Here's how the part is built. I have some questions about the finished solid (model axes, mm). A direction names the side the tool comes from. Give positions to 0.01 mm unless a question says otherwise; leave off trailing zeros. Write each loop counter-clockwise with the first axis right and the second up, starting at its lowest first coordinate (ties: lowest second). Pieces come first, ordered by that corner, then holes. Notation, with made-up numbers: (85.25, 0.25) -> (91.25, 0.25) arc R30 ccw to (91.25, 37.25) -> close; hole circle Ø6 at (59, 61). An arc over 180 degrees is marked (long way). Return JSON: item names as keys, results as strings.
from build123d import *

# Parameters (mm, degrees)
F0_W     = 38.1
F0_H     = 25.4
F1_DEPTH = 12.7
F2_W     = 34.925
F2_H     = 22.225
F3_DEPTH = 1.5875
F4_R     = 0.762
F5_R     = 0.254


with BuildPart() as f1:
    # F0 (on Top) → F1 (new body)
    with BuildSketch(Plane.XY):
        Rectangle(F0_W, F0_H)
    extrude(amount=F1_DEPTH)

    # F2 (on face) → F3 (cut)
    with BuildSketch(Plane.XY.offset(12.7)):
        Rectangle(F2_W, F2_H)
    extrude(amount=-F3_DEPTH, mode=Mode.SUBTRACT)

    # F4
    f4_edges = [f1.edges().sort_by_distance(p)[0] for p in [
        (-19.05, -12.7, 6.35),
        (-19.05, 12.7, 6.35),
        (19.05, 12.7, 6.35),
        (19.05, -12.7, 6.35),
    ]]
    fillet(f4_edges, radius=F4_R)

    # F5
    f5_edges = [f1.edges().sort_by_distance(p)[0] for p in [
        (0, 12.7, 12.7),
        (18.826815, 12.476815, 12.7),
        (-18.826815, 12.476815, 12.7),
        (19.05, 0, 12.7),
        (-19.05, 0, 12.7),
        (18.826815, -12.476815, 12.7),
        (-18.826815, -12.476815, 12.7),
        (0, -12.7, 12.7),
        (0, 11.1125, 12.7),
        (-17.4625, 0, 12.7),
        (0, -11.1125, 12.7),
        (17.4625, 0, 12.7),
    ]]
    fillet(f5_edges, radius=F5_R)


solid = f1.part
1. Which directions (+Z, -Z, +X, -X, +Y, -Y) give clear straight access to the entire face, cutting with the end or side of a thin tool? Please do faces 1 (the face through (0, 0, 0)), 2 (the face through (0, 11.112, 12)).
Taken from the geometry:
{"face 1": "-Z, +X, -X, +Y, -Y", "face 2": "+Z"}
2. Suppose I cut it at A-A, the plane y = 2.25. List the corners of the cut face in (x, z) for me, and give its area (3 significant figures).
Taken from the geometry:
{"outline": "(-19.05, 0) -> (19.05, 0) -> (19.05, 12.45) arc R0.25 ccw to (18.8, 12.7) -> (17.72, 12.7) arc R0.25 ccw to (17.46, 12.45) -> (17.46, 11.11) -> (-17.46, 11.11) -> (-17.46, 12.45) arc R0.25 ccw to (-17.72, 12.7) -> (-18.8, 12.7) arc R0.25 ccw to (-19.05, 12.45) -> close", "area": "428 mm²"}
3. Suppose I cut it at B-B, the plane z = 12. List the corners of the cut face in (x, y) for me.
Taken from the geometry:
{"outline": "(-19.05, -11.94) arc R0.76 ccw to (-18.29, -12.7) -> (18.29, -12.7) arc R0.76 ccw to (19.05, -11.94) -> (19.05, 11.94) arc R0.76 ccw to (18.29, 12.7) -> (-18.29, 12.7) arc R0.76 ccw to (-19.05, 11.94) -> close; hole (-17.46, -11.11) -> (17.46, -11.11) -> (17.46, 11.11) -> (-17.46, 11.11) -> close"}
4. For pin 1 Ø6.5 at (x, y) = (-7, -0.5) entering from +Z, with a flat end and sliding along its axis, tell me the tip position at first contact or that it passes through.
Taken from the geometry:
{"pin 1": "stops at z = 11.11"}
5. If I drill on line 1 (Y direction, x = 2, z = 12); line 2 (X direction, y = -1.75, z = 11.5); line 3 (Z direction, x = 9, y = 8.25), over which ranges is the centre line in solid material (lowest first)? Write a range as [from, to].
Taken from the geometry:
{"line 1": "y = [-12.7, -11.11], [11.11, 12.7]", "line 2": "x = [-19.05, -17.46], [17.46, 19.05]", "line 3": "z = [0, 11.11]"}
6. If we mould it in two halves opening along X, with no side actions, what happens to faces 3 (the face through (17.462, 0, 12)), 4 (the face through (0, 12.7, 6)), 5 (the face through (19.05, 0, 6))? For each: released by +X, released by -X, zero draft, split by the parting line, or undercut.
Taken from the geometry:
{"face 3": "undercut", "face 4": "zero draft", "face 5": "released by +X"}
7. Suppose I cut it at C-C, the plane x = 8. List the corners of the cut face in (y, z) for me, and give its area (3 significant figures).
Taken from the geometry:
{"outline": "(-12.7, 0) -> (12.7, 0) -> (12.7, 12.45) arc R0.25 ccw to (12.45, 12.7) -> (11.37, 12.7) arc R0.25 ccw to (11.11, 12.45) -> (11.11, 11.11) -> (-11.11, 11.11) -> (-11.11, 12.45) arc R0.25 ccw to (-11.37, 12.7) -> (-12.45, 12.7) arc R0.25 ccw to (-12.7, 12.45) -> close", "area": "287 mm²"}
